Answer from the drawing. Dimensions are ordinates in mm from the lowest x, y and z of the part. Give positions to 0.01 mm unless a question says otherwise; leave off trailing zeros. Order: outer loops, then holes, each group sorted by start corner. A loop starts at its lowest first (then second) coordinate and runs counter-clockwise, first axis right, second up. Notation, with made-up numbers: (20, 53.5) - (26, 53.5) arc R14 ccw to (26, 61.5) - close; hole circle Ø6 at (-35, 39). An arc over 180 degrees is marked (long way). Write each question's results on one line, items separated by ' | '.
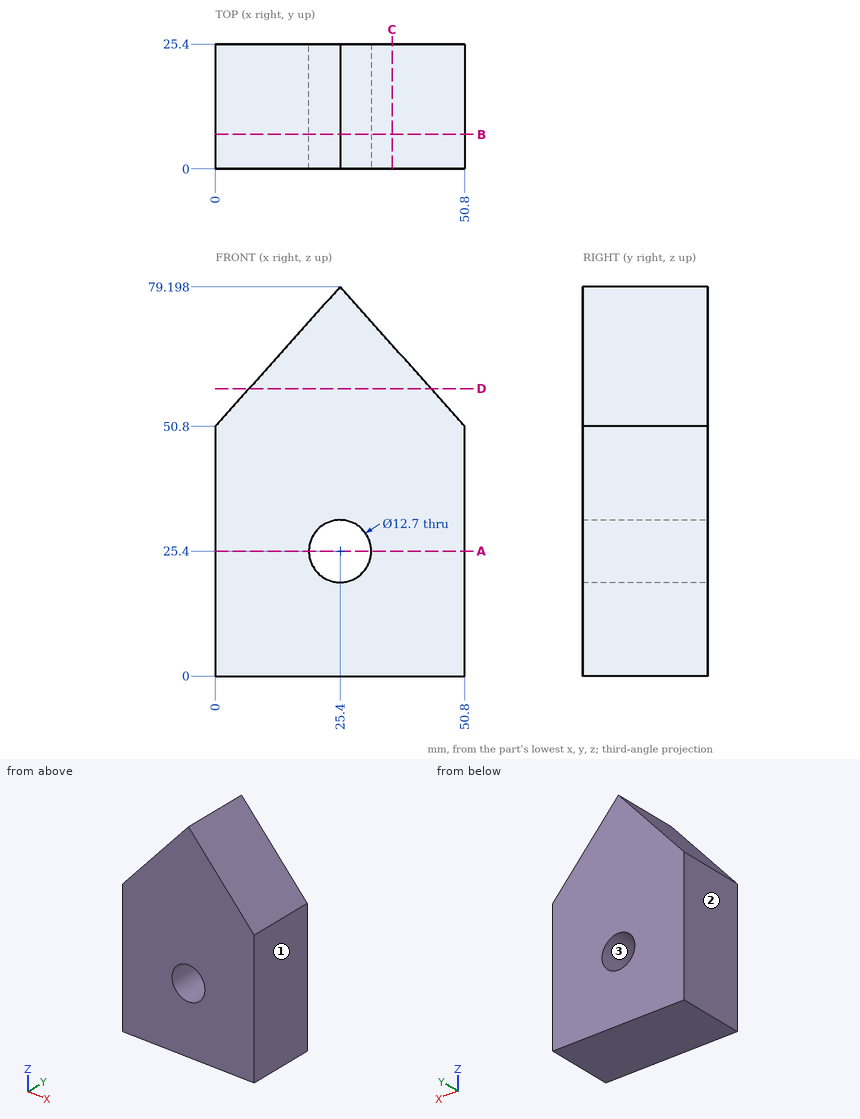
1. Determine the mould class of the marked faces 1, 2 and 3 for opening direction X: +X half, -X half, draft (parallel to the pull), parting line (faces both ways), or undercut.
Answer list:
face 1: +X half | face 2: -X half | face 3: undercut
2. Straight lines are drawn through the part: line 1 (X direction, y = 1.5, z = 20); line 2 (Z direction, x = 23, y = 22.75) (1 decimal); line 3 (X direction, y = 2, z = 31). For each, find the intervals that lie inside material, in ascending order. Write a range as [from, to].
Answer list:
line 1: [0, 22.06], [28.74, 50.8] | line 2: [0, 19.5], [31.3, 76.5] | line 3: [0, 22.41], [28.39, 50.8]
3. A cutting plane is placed at C-C, the plane x = 36. Write down the section's boundary in (y, z).
Answer list:
outline: (0, 0) - (25.4, 0) - (25.4, 67.35) - (0, 67.35) - close
4. Given P1, Ø4, axis at y = 20.5, z = 62.5, coming from the +X side; P2, Ø10, axis at x = 34, y = 22.5, coming from the +Z side; P3, Ø4, axis at x = 33.5, y = 11, coming from the +Z side, each flat-ended and moving along its own axis, determine where each tip first touches the part or whether it passes through.
Answer list:
P1: x = 42.12 | P2: z = 75.17 | P3: z = 72.38
5. A cutting plane is placed at A-A, the plane z = 25.4. Write down the section's boundary in (x, y).
Answer list:
outline: (0, 0) - (19.05, 0) - (19.05, 25.4) - (0, 25.4) - close; (31.75, 0) - (50.8, 0) - (50.8, 25.4) - (31.75, 25.4) - close
6. A cutting plane is placed at B-B, the plane y = 7. Write down the section's boundary in (x, z).
Answer list:
outline: (0, 0) - (50.8, 0) - (50.8, 50.8) - (25.4, 79.2) - (0, 50.8) - close; hole circle Ø12.7 at (25.4, 25.4)
7. A cutting plane is placed at D-D, the plane z = 58.5. Write down the section's boundary in (x, y), then the cut area to 3 significant figures.
Answer list:
outline: (6.89, 0) - (43.91, 0) - (43.91, 25.4) - (6.89, 25.4) - close | area: 940 mm^2
